```python
from build123d import *

# Parameters (mm, degrees)
F0_W     = 101.6
F0_H     = 6.35
F3_DEPTH = 13.97
F4_DEPTH = 2.794


with BuildPart() as f1:
    # F0 (on Front) → F1 (revolve)
    with BuildSketch(Plane.XZ):
        with Locations((0, -3.175)):
            Rectangle(F0_W, F0_H)
    revolve(axis=Axis((-107.179771, 0, 0), (-1, 0, 0)))

    # F2 (on face) → F3 (join)
    with BuildSketch(Plane.YZ.offset(50.8)):
        with BuildLine():
            ThreePointArc((31.75, 0), (38.1, 6.35), (44.45, 0))
            Line((44.45, 0), (50.8, 0))
            ThreePointArc((50.8, 0), (19.05, 31.75), (-12.7, 0))
            Line((-12.7, 0), (31.75, 0))
        make_face()
        with BuildLine():
            Line((50.8, 0), (44.45, 0))
            ThreePointArc((44.45, 0), (38.1, -6.35), (31.75, 0))
            Line((31.75, 0), (-12.7, 0))
            ThreePointArc((-12.7, 0), (19.05, -31.75), (50.8, 0))
        make_face()
    extrude(amount=F3_DEPTH)


with BuildPart() as f4:
    # F2 (on face) → F4 (new body)
    with BuildSketch(Plane.YZ.offset(50.8)):
        with BuildLine():
            Line((50.8, 0), (44.45, 0))
            ThreePointArc((44.45, 0), (38.1, -6.35), (31.75, 0))
            Line((31.75, 0), (6.35, 0))
            ThreePointArc((6.35, 0), (0, -6.35), (-6.35, 0))
            Line((-6.35, 0), (-12.7, 0))
            ThreePointArc((-12.7, 0), (19.05, -31.75), (50.8, 0))
        make_face()
        with BuildLine():
            ThreePointArc((31.75, 0), (38.1, 6.35), (44.45, 0))
            Line((44.45, 0), (50.8, 0))
            ThreePointArc((50.8, 0), (19.05, 31.75), (-12.7, 0))
            Line((-12.7, 0), (-6.35, 0))
            ThreePointArc((-6.35, 0), (0, 6.35), (6.35, 0))
            Line((6.35, 0), (31.75, 0))
        make_face()
    extrude(amount=F4_DEPTH)


solid = f1.part
```
Geometry check sheet. Reference: the model listing, model coordinates, mm. Round coordinates to 2 decimals unless told otherwise and drop trailing zeros. Loops run counter-clockwise (first coordinate to the right, second up) from the corner with the lowest first, then second, coordinate; pieces in that order, holes last. Notation, with made-up numbers: (69.5, 29) - (103.5, 29) arc R26 ccw to (103.5, 62) - close; hole circle Ø1 at (-36.5, 79). An arc over 180 degrees is marked (long way). Use a Markdown table: item, result.
Q1. Cross-section at B-B on z = 0. Record the cut outline in (x, y), plus the area to 3 significant figures.
Solutions:
| item | result |
|---|---|
| outline | (-50.8, -6.35) - (50.8, -6.35) - (50.8, -12.7) - (64.77, -12.7) - (64.77, 31.75) - (50.8, 31.75) - (50.8, 6.35) - (-50.8, 6.35) - close; (50.8, 44.45) - (64.77, 44.45) - (64.77, 50.8) - (50.8, 50.8) - close |
| area | 2,000 mm2 |
Q2. Cross-section at A-A on y = 38.1. Record the cut outline in (x, z).
Solutions:
| item | result |
|---|---|
| outline | (50.8, -25.4) - (64.77, -25.4) - (64.77, -6.35) - (50.8, -6.35) - close; (50.8, 6.35) - (64.77, 6.35) - (64.77, 25.4) - (50.8, 25.4) - close |
Q3. Cross-section at C-C on y = 3. Record the cut outline in (x, z).
Solutions:
| item | result |
|---|---|
| outline | (-50.8, -5.6) - (50.8, -5.6) - (50.8, -27.39) - (64.77, -27.39) - (64.77, 27.39) - (50.8, 27.39) - (50.8, 5.6) - (-50.8, 5.6) - close |
Q4. Material ranges on line 1 (X direction, y = -6, z = -19); line 2 (Z direction, x = 59, y = 38); line 3 (Z direction, x = 56, y = 38.1), recorded low to high.
Solutions:
| item | result |
|---|---|
| line 1 | x = 50.8 to 64.77 |
| line 2 | z = -25.47 to -6.35, 6.35 to 25.47 |
| line 3 | z = -25.4 to -6.35, 6.35 to 25.4 |
Q5. Go/stop test with flat-tipped pins: P1, Ø5, axis at x = -37, y = 2.5, coming from the -Z side; P2, Ø4, axis at y = 38.5, z = 18, coming from the -X side; P3, Ø1, axis at x = -24, z = -6, coming from the -Y side. Record where each tip stops, or that it passes through.
Solutions:
| item | result |
|---|---|
| P1 | stops at z = -6.35 |
| P2 | stops at x = 50.8 |
| P3 | stops at y = -3.17 |
Q6. Cross-section at D-D on x = -18. Record the cut outline in (y, z), plus the area to 3 significant figures.
Solutions:
| item | result |
|---|---|
| outline | circle Ø12.7 at (0, 0) |
| area | 127 mm2 |
Q7. Draft check along Z on faces 1 (the flat face through (50.8, 19, 0)), 2 (the cylindrical face through (57.687, 31.756, -0.279)), 3 (the cylindrical face through (0.71, 6.2, 1.38)). Enter one of: released by +Z, released by -Z, zero draft, split by the parting line, or undercut.
Solutions:
| item | result |
|---|---|
| face 1 | zero draft |
| face 2 | undercut |
| face 3 | split by the parting line |
